Can you work these out from the model? Positions are in its coordinate system, mm. A direction names the side the tool comes from. Coordinates: 2 decimals unless noted, no trailing zeros. Order: outer loops, then holes, each group sorted by start corner. A loop starts at its lowest first (then second) coordinate and runs counter-clockwise, first axis right, second up. Notation, with made-up numbers: (75.5, -39.75) - (122.5, -39.75) arc R17 cw to (122.5, -19.75) - close; hole circle Ø11 at (34.5, 73.25). An arc over 180 degrees is marked (long way). Use a Markdown table: item, result. Add a question column.
(1) On a 3-axis mill with a long thin cutter (end or side, diameter ignored), from which of +Z, -Z, +X, -X, +Y, -Y can I reach the whole of each face in a straight line? I mean faces 1 (the cylindrical face through (40.524, -0.47, -3.889)), 2 (the flat face through (50, -2, -63.5)), 3 (the flat face through (14, -2, 0)). Say none if no direction works.
(2) I want a section at A-A (z = -31.75). List the corners of the cut face in (x, y) for me (1 decimal), and give its area (3 significant figures).
(3) We'd pull the mould along Z, two halves only. Please class faces 4 (the cylindrical face through (2.037, -1.891, -61.352)), 5 (the cylindrical face through (2.148, -1.891, -2.037)), 6 (the flat face through (63.5, -2, -50)), 7 (the cylindrical face through (53.7, -0.47, -17.75)): pulls with the +Z half, pulls with the -Z half, needs draft (parallel to the pull), parting line crosses it, or undercut.
(4) If I drill on L1, parallel to X at y = -0.25, z = -31.75 (3 decimals); L2, parallel to X at y = -2.7, z = -8.5; L3, parallel to Z at x = 55.5, y = -0.7, over which ranges is the centre line in solid material (lowest first)? Write a range as [from, to].
(5) I want a section at C-C (y = -2.55). State how many separate pieces and enclosed holes the cut face has, and give its area (3 significant figures).
(6) For pin 1 Ø4.5 at (x, z) = (56.36, -56.36) entering from -Y; pin 2 Ø1.9 at (y, z) = (-2, -50.5) entering from +X; pin 3 Ø1.9 at (x, y) = (15.5, -3) entering from +Z; pin 4 Ø1.2 at (y, z) = (-2.5, -48.5) entering from -X, each with a flat end and sliding along its axis, tell me the tip position at first contact or that it passes through.
(7) I want a section at B-B (x = 31.75). List the corners of the cut face in (y, z) for me (1 decimal).
```python
from build123d import *

# Parameters (mm, degrees)
SKETCH1_R           = 22.1742
SKETCH1_R_2         = 2.38125
BOSS_EXTRUDE1_DEPTH = 3.8354
SKETCH2_R           = 29.21
SKETCH2_R_2         = 26.035
CUT_EXTRUDE1_DEPTH  = 0.9525


with BuildPart() as part:
    # Sketch1 → Boss-Extrude1 (new body)
    with BuildSketch(Plane(origin=(0, 0, 0), x_dir=(1, 0, 0), z_dir=(0, 1, 0))):
        with BuildLine():
            Line((0, 43.62908334), (0, 56.35625))
            ThreePointArc((0, 56.35625), (2.092355932, 61.407644068), (7.14375, 63.5))
            Line((7.14375, 63.5), (19.87091666, 63.5))
            ThreePointArc((19.87091666, 63.5), (21.269548228, 63.596728676), (22.641548343, 63.885072886))
            ThreePointArc((22.641548343, 63.885072886), (31.75, 65.151), (40.858451657, 63.885072886))
            ThreePointArc((40.858451657, 63.885072886), (42.230451772, 63.596728676), (43.62908334, 63.5))
            Line((43.62908334, 63.5), (56.35625, 63.5))
            ThreePointArc((56.35625, 63.5), (61.407644068, 61.407644068), (63.5, 56.35625))
            Line((63.5, 56.35625), (63.5, 43.62908334))
            ThreePointArc((63.5, 43.62908334), (63.596728676, 42.230451772), (63.885072886, 40.858451657))
            ThreePointArc((63.885072886, 40.858451657), (65.151, 31.75), (63.885072886, 22.641548343))
            ThreePointArc((63.885072886, 22.641548343), (63.596728676, 21.269548228), (63.5, 19.87091666))
            Line((63.5, 19.87091666), (63.5, 7.14375))
            ThreePointArc((63.5, 7.14375), (61.407644068, 2.092355932), (56.35625, 0))
            Line((56.35625, 0), (43.62908334, 0))
            ThreePointArc((43.62908334, 0), (42.230451772, -0.096728676), (40.858451657, -0.385072886))
            ThreePointArc((40.858451657, -0.385072886), (31.75, -1.651), (22.641548343, -0.385072886))
            ThreePointArc((22.641548343, -0.385072886), (21.269548228, -0.096728676), (19.87091666, 0))
            Line((19.87091666, 0), (7.14375, 0))
            ThreePointArc((7.14375, 0), (2.092355932, 2.092355932), (0, 7.14375))
            Line((0, 7.14375), (0, 19.87091666))
            ThreePointArc((0, 19.87091666), (-0.096728676, 21.269548228), (-0.385072886, 22.641548343))
            ThreePointArc((-0.385072886, 22.641548343), (-1.651, 31.75), (-0.385072886, 40.858451657))
            ThreePointArc((-0.385072886, 40.858451657), (-0.096728676, 42.230451772), (0, 43.62908334))
        make_face()
        with Locations(Location((31.75, 31.75, 0), (0, 0, 270))):
            Circle(SKETCH1_R, mode=Mode.SUBTRACT)
        with Locations(Location((56.35625, 56.35625, 0), (0, 0, 270))):
            Circle(SKETCH1_R_2, mode=Mode.SUBTRACT)
        with Locations(Location((56.35625, 7.14375, 0), (0, 0, 270))):
            Circle(SKETCH1_R_2, mode=Mode.SUBTRACT)
        with Locations(Location((7.14375, 7.14375, 0), (0, 0, 270))):
            Circle(SKETCH1_R_2, mode=Mode.SUBTRACT)
        with Locations(Location((7.14375, 56.35625, 0), (0, 0, 270))):
            Circle(SKETCH1_R_2, mode=Mode.SUBTRACT)
    extrude(amount=-BOSS_EXTRUDE1_DEPTH)

    # Sketch2 → Cut-Extrude1 (cut)
    with BuildSketch(Plane(origin=(0, 0, 0), x_dir=(1, 0, 0), z_dir=(0, 1, 0))):
        with Locations(Location((31.75, 31.75, 0), (0, 0, 270))):
            Circle(SKETCH2_R)
        with Locations(Location((31.75, 31.75, 0), (0, 0, 270))):
            Circle(SKETCH2_R_2, mode=Mode.SUBTRACT)
    extrude(amount=-CUT_EXTRUDE1_DEPTH, mode=Mode.SUBTRACT)


solid = part.part
```
Answers follow:
| question | item | result |
|---|---|---|
| 1 | face 1 | +Y |
| 1 | face 2 | -Z, +X, +Y, -Y |
| 1 | face 3 | +Z, -X, +Y, -Y |
| 2 | outline | (-1.7, -3.8) - (9.6, -3.8) - (9.6, 0) - (5.7, 0) - (5.7, -1) - (2.5, -1) - (2.5, 0) - (-1.7, 0) - close; (53.9, -3.8) - (65.2, -3.8) - (65.2, 0) - (61, 0) - (61, -1) - (57.8, -1) - (57.8, 0) - (53.9, 0) - close |
| 2 | area | 80.1 mm² |
| 3 | face 4 | pulls with the -Z half |
| 3 | face 5 | pulls with the +Z half |
| 3 | face 6 | needs draft |
| 3 | face 7 | undercut |
| 4 | L1 | x = [-1.651, 2.54], [5.715, 9.576], [53.924, 57.785], [60.96, 65.151] |
| 4 | L2 | x = [0, 5.19], [9.1, 54.4], [58.31, 63.5] |
| 4 | L3 | z = [-63.5, -58.58], [-54.13, -48.75], [-42.42, -21.08], [-14.75, -9.37], [-4.92, 0] |
| 5 | separate pieces | 1 |
| 5 | enclosed holes | 5 |
| 5 | area | 2,470 mm² |
| 6 | pin 1 | passes through |
| 6 | pin 2 | stops at x = 63.5 |
| 6 | pin 3 | stops at z = 0 |
| 6 | pin 4 | stops at x = 0 |
| 7 | outline | (-3.8, -65.2) - (0, -65.2) - (0, -61) - (-1, -61) - (-1, -57.8) - (0, -57.8) - (0, -53.9) - (-3.8, -53.9) - close; (-3.8, -9.6) - (0, -9.6) - (0, -5.7) - (-1, -5.7) - (-1, -2.5) - (0, -2.5) - (0, 1.7) - (-3.8, 1.7) - close |
